Can you work these out from the model? Positions are in its coordinate system, mm. A direction names the side the tool comes from. Give positions to 0.01 mm unless a question says otherwise; leave off trailing zeros. Order: outer loops, then holes, each group sorted by start corner. A loop starts at its lowest first (then second) coordinate and runs counter-clockwise, first axis right, second up. Notation, with made-up numbers: (-31.75, 20.25) -> (-22.75, 20.25) arc R36 ccw to (-22.75, 55.25) -> close; hole circle Ø10 at (61.5, 76.5). An arc over 180 degrees is marked (long way). Answer as a JSON object with one key per item and string values.
```python
from build123d import *

# Parameters (mm, degrees)
ESBO_O1_R                 = 25.25
RESSALTO_EXTRUS_O1_DEPTH  = 35
ESBO_O2_R                 = 20
RESSALTO_EXTRUS_O2_DEPTH  = 54
ESBO_O3_R                 = 14.25
RESSALTO_EXTRUS_O3_DEPTH  = 1.5
FURO_ROSCADO_DE_M41_D     = 3.3
FURO_ROSCADO_DE_M41_DEPTH = 11.5
FURO_ROSCADO_DE_M41_TIP   = 0.991420021
ESBO_O7_R                 = 3.15
RESSALTO_EXTRUS_O4_DEPTH  = 18
CHANFRO1_SIZE             = 0.25
ESBO_O8_R                 = 2
RESSALTO_EXTRUS_O5_DEPTH  = 15
CHANFRO2_SIZE             = 0.5
ESBO_O9_R                 = 6
ESBO_O9_R_2               = 2.25
RESSALTO_EXTRUS_O6_DEPTH  = 1
CHANFRO3_SIZE             = 0.5
ESBO_O10_W                = 33
ESBO_O10_H                = 15.540446693


with BuildPart() as part:
    # Esboço1 → Ressalto-extrusão1 (new body)
    with BuildSketch(Plane.XY):
        Circle(ESBO_O1_R)
    extrude(amount=RESSALTO_EXTRUS_O1_DEPTH)

    # Esboço2 → Ressalto-extrusão2 (add)
    with BuildSketch(Plane.XY.offset(35)):
        Circle(ESBO_O2_R)
    extrude(amount=RESSALTO_EXTRUS_O2_DEPTH)

    # Esboço3 → Ressalto-extrusão3 (add)
    with BuildSketch(Plane(origin=(0, 0, 0), x_dir=(-1, 0, 0), z_dir=(0, 0, -1))):
        with Locations(Location((0, 0, 0), (0, 0, 180))):
            Circle(ESBO_O3_R)
    extrude(amount=RESSALTO_EXTRUS_O3_DEPTH)

    # Furo roscado de M41
    with Locations(Plane(origin=(0, 0, 0), x_dir=(-1, 0, 0), z_dir=(0, 0, -1))):
        with Locations((-19, 0), (19, 0)):
            Hole(FURO_ROSCADO_DE_M41_D / 2, depth=FURO_ROSCADO_DE_M41_DEPTH)
            with Locations((0, 0, -(FURO_ROSCADO_DE_M41_DEPTH + FURO_ROSCADO_DE_M41_TIP / 2))):  # 118° drill point
                Cone(0, FURO_ROSCADO_DE_M41_D / 2, FURO_ROSCADO_DE_M41_TIP, mode=Mode.SUBTRACT)

    # Esboço7 → Ressalto-extrusão4 (add)
    with BuildSketch(Plane(origin=(0, 0, -1.5), x_dir=(-1, 0, 0), z_dir=(0, 0, -1))):
        with Locations((0, 8.5)):
            Circle(ESBO_O7_R)
    extrude(amount=RESSALTO_EXTRUS_O4_DEPTH)

    # Chanfro1
    chanfro1_edges = [part.edges().sort_by_distance(p)[0] for p in [
        (3.15, 8.5, -19.5),
    ]]
    chamfer(chanfro1_edges, length=CHANFRO1_SIZE)

    # Esboço8 → Ressalto-extrusão5 (add)
    with BuildSketch(Plane.XY.offset(89)):
        Circle(ESBO_O8_R)
    extrude(amount=RESSALTO_EXTRUS_O5_DEPTH)

    # Chanfro2
    chanfro2_edges = [part.edges().sort_by_distance(p)[0] for p in [
        (-2, 0, 104),
    ]]
    chamfer(chanfro2_edges, length=CHANFRO2_SIZE)

    # Esboço9 → Ressalto-extrusão6 (add)
    with BuildSketch(Plane.XY.offset(89)):
        Circle(ESBO_O9_R)
        Circle(ESBO_O9_R_2, mode=Mode.SUBTRACT)
    extrude(amount=RESSALTO_EXTRUS_O6_DEPTH)

    # Chanfro3
    chanfro3_edges = [part.edges().sort_by_distance(p)[0] for p in [
        (-6, 0, 90),
    ]]
    chamfer(chanfro3_edges, length=CHANFRO3_SIZE)

    # Esboço10 → Corte-Revolução1 (revolve, cut)
    with BuildSketch(Plane(origin=(0, 0, 0), x_dir=(0, 0, -1), z_dir=(1, 0, 0)), mode=Mode.PRIVATE) as corte_revolu_o1_sk:
        with Locations((-17.5, 32.770223347)):
            Rectangle(ESBO_O10_W, ESBO_O10_H)
    revolve(corte_revolu_o1_sk.sketch.rotate(Axis((0, 0, 0), (0, 0, 1)), 90), axis=Axis((0, 0, 0), (0, 0, 1)), mode=Mode.SUBTRACT)


solid = part.part
```
1. If we section it at C-C on y = -10: Please give me the cut outline in (x, z), then the cut area to 3 significant figures.
Worked answers:
{"outline": "(-23.19, 0) -> (-10.15, 0) -> (-10.15, -1.5) -> (10.15, -1.5) -> (10.15, 0) -> (23.19, 0) -> (23.19, 1) -> (22.91, 1) -> (22.91, 34) -> (23.19, 34) -> (23.19, 35) -> (17.32, 35) -> (17.32, 89) -> (-17.32, 89) -> (-17.32, 35) -> (-23.19, 35) -> (-23.19, 34) -> (-22.91, 34) -> (-22.91, 1) -> (-23.19, 1) -> close", "area": "3,510 mm²"}
2. Please list where these lines run through material, in increasing order: L1, parallel to Y at x = 0, z = 89.75; L2, parallel to Z at x = 13, y = 17; L3, parallel to Z at x = 17.5, y = -6.5.
Worked answers:
{"L1": "-5.75 to -2.25, -2 to 2, 2.25 to 5.75", "L2": "0 to 35", "L3": "0 to 89"}
3. Will these pins go through, and if not, where does the flat tip stop? pin 1 Ø8 at (y, z) = (17, 7.5) entering from +X; pin 2 Ø15 at (x, y) = (-7, -4) entering from -Z; pin 3 Ø3 at (x, z) = (-6, 58.5) entering from +Y; pin 4 Ø5.5 at (x, y) = (-0.5, 2.5) entering from +Z.
Worked answers:
{"pin 1": "x = 21.35", "pin 2": "z = -1.5", "pin 3": "y = 19.49", "pin 4": "z = 104"}
4. If we section it at A-A on y = 22: Please give me the cut outline in (x, z).
Worked answers:
{"outline": "(-12.39, 0) -> (12.39, 0) -> (12.39, 1) -> (11.87, 1) -> (11.87, 34) -> (12.39, 34) -> (12.39, 35) -> (-12.39, 35) -> (-12.39, 34) -> (-11.87, 34) -> (-11.87, 1) -> (-12.39, 1) -> close"}
5. If we section it at B-B on z = 55.5: Please give me the cut outline in (x, y), then the cut area to 3 significant figures.
Worked answers:
{"outline": "circle Ø40 at (0, 0)", "area": "1,260 mm²"}
6. For faces 1 (the face through (-4.336, -19.524, 61.622)), 2 (the face through (0, 9, -19.5)), 3 (the face through (0.41, 11.623, -10.251)), which set-ups out of +Z, -Z, +X, -X, +Y, -Y let a thin tool reach every point of the face, with its end or its side?
Worked answers:
{"face 1": "+Z", "face 2": "-Z, +X, -X, +Y, -Y", "face 3": "-Z"}
7. If we section it at D-D on z = 27: Please give me the cut outline in (x, y).
Worked answers:
{"outline": "circle Ø50 at (0, 0)"}
8. If we mould it in two halves opening along X, with no side actions, what happens to faces 4 (the face through (-19.3, -0.1, 12.3)), 5 (the face through (-5.994, 0.264, 89.246)), 6 (the face through (-0.1, -2.4, 90)), 7 (the face through (17.69, -1, 5.83))? For each: +X half, -X half, draft (parallel to the pull), parting line (faces both ways), or undercut.
Worked answers:
{"face 4": "undercut", "face 5": "parting line", "face 6": "draft", "face 7": "undercut"}
